Here's how the part is built. I have some questions about the finished solid (model axes, mm). A direction names the side the tool comes from. Give positions to 0.01 mm unless a question says otherwise; leave off trailing zeros. Loops run counter-clockwise (first coordinate to the right, second up) from the corner with the lowest first, then second, coordinate; pieces in that order, holes last. Notation, with made-up numbers: (79.25, -39.5) - (138.25, -39.5) arc R24 cw to (138.25, -6.5) - close; hole circle Ø8 at (32, 20). An arc over 180 degrees is marked (long way). Use one line per item in the form item = value.
from build123d import *

# Parameters (mm, degrees)
SKETCH1_W           = 34.925
SKETCH1_H           = 25.4
BOSS_EXTRUDE1_DEPTH = 1.5875
BOSS_EXTRUDE2_DEPTH = 4.7625
SKETCH4_W           = 14.2875
SKETCH4_H           = 9.525
BOSS_EXTRUDE7_DEPTH = 6.35
SKETCH6_R           = 1.190625
CUT_EXTRUDE1_DEPTH  = 24.759524406


with BuildPart() as part:
    # Sketch1 → Boss-Extrude1 (new body)
    with BuildSketch(Plane(origin=(0, 0, 0), x_dir=(1, 0, 0), z_dir=(0, 1, 0))):
        Rectangle(SKETCH1_W, SKETCH1_H)
    extrude(amount=BOSS_EXTRUDE1_DEPTH)

    # Sketch2 → Boss-Extrude2 (add)
    with BuildSketch(Plane(origin=(0, 1.5875, 0), x_dir=(1, 0, 0), z_dir=(0, 1, 0))):
        Polygon((-4.7625, 11.1125), (11.1125, 11.1125), (11.1125, 6.35), (17.4625, 6.35), (17.4625, -6.35), (11.1125, -6.35), (11.1125, -11.1125), (-4.7625, -11.1125), align=None)
    extrude(amount=BOSS_EXTRUDE2_DEPTH)

    # Sketch4 → Boss-Extrude7 (add)
    with BuildSketch(Plane(origin=(0, 1.5875, 0), x_dir=(1, 0, 0), z_dir=(0, 1, 0))):
        with Locations((-11.90625, 0)):
            Rectangle(SKETCH4_W, SKETCH4_H)
    extrude(amount=BOSS_EXTRUDE7_DEPTH)

    # Sketch6 → Cut-Extrude1 (cut, through all)
    with BuildSketch(Plane(origin=(0, 1.5875, 0), x_dir=(1, 0, 0), z_dir=(0, 1, 0))):
        with Locations(Location((-15.875, 11.1125, 0), (0, 0, 270))):
            Circle(SKETCH6_R)
        with Locations(Location((-15.875, -11.1125, 0), (0, 0, 270))):
            Circle(SKETCH6_R)
        with Locations(Location((15.875, -11.1125, 0), (0, 0, 270))):
            Circle(SKETCH6_R)
        with Locations(Location((15.875, 11.1125, 0), (0, 0, 270))):
            Circle(SKETCH6_R)
    extrude(amount=-CUT_EXTRUDE1_DEPTH, mode=Mode.SUBTRACT)


solid = part.part
(1) If I drill on probe 1 along Y at (x, z) = (4, 6.25); probe 2 along Z at (x, y) = (0, 5.5); probe 3 along X at (y, z) = (7.5, -4.5), over which ranges is the centre line in solid material (lowest first)?
Geometry says:
probe_1 = 0 to 6.35
probe_2 = -11.11 to 11.11
probe_3 = -19.05 to -4.76
(2) For faces 1 (the flat face through (14, 4, -6.35)), 2 (the flat face through (-17.462, 1, 0)), 3 (the flat face through (3, 4, -11.112)), which set-ups out of +Z, -Z, +X, -X, +Y, -Y let a thin tool reach every point of the face, with its end or its side?
Geometry says:
face_1 = -Z, +X, +Y
face_2 = +Z, -Z, -X, -Y
face_3 = -Z, +X, -X, +Y
(3) For P1, Ø1.3, axis at x = -18, z = -2, coming from the -Y side; P2, Ø4, axis at y = 4.5, z = -8.5, coming from the +X side; P3, Ø3, axis at x = 15.88, z = 11.11, coming from the +Y side; P4, Ø4, axis at x = 5.5, z = -7.5, coming from the +Y side, each with a flat end and sliding along its axis, tell me the tip position at first contact or that it passes through.
Geometry says:
P1 = 0
P2 = 11.11
P3 = 1.59
P4 = 6.35
(4) Thinking about a two-plate mould opening in Z: for faces 4 (the flat face through (0, 1, 12.7)), 5 (the cylindrical face through (17.055, 0.805, 10.958)), 6 (the flat face through (-12, 5, -4.762)), which applies, pulls with the +Z half, pulls with the -Z half, needs draft (parallel to the pull), parting line crosses it, or undercut?
Geometry says:
face_4 = pulls with the +Z half
face_5 = undercut
face_6 = pulls with the -Z half
(5) If we section it at C-C (y = 5): List the corners of the cut face in (x, z) for me.
Geometry says:
outline = (-19.05, -4.76) - (-4.76, -4.76) - (-4.76, -11.11) - (11.11, -11.11) - (11.11, -6.35) - (17.46, -6.35) - (17.46, 6.35) - (11.11, 6.35) - (11.11, 11.11) - (-4.76, 11.11) - (-4.76, 4.76) - (-19.05, 4.76) - close
(6) If we section it at D-D (x = 15.5): List the corners of the cut face in (y, z) for me.
Geometry says:
outline = (0, -12.7) - (1.59, -12.7) - (1.59, -12.24) - (0, -12.24) - close; (0, -9.98) - (1.59, -9.98) - (1.59, -6.35) - (6.35, -6.35) - (6.35, 6.35) - (1.59, 6.35) - (1.59, 9.98) - (0, 9.98) - close; (0, 12.24) - (1.59, 12.24) - (1.59, 12.7) - (0, 12.7) - close
(7) If we section it at B-B (z = -8.25): List the corners of the cut face in (x, y) for me.
Geometry says:
outline = (-17.46, 0) - (17.46, 0) - (17.46, 1.59) - (11.11, 1.59) - (11.11, 6.35) - (-4.76, 6.35) - (-4.76, 1.59) - (-17.46, 1.59) - close
(8) If we section it at A-A (x = 5.5): List the corners of the cut face in (y, z) for me.
Geometry says:
outline = (0, -12.7) - (1.59, -12.7) - (1.59, -11.11) - (6.35, -11.11) - (6.35, 11.11) - (1.59, 11.11) - (1.59, 12.7) - (0, 12.7) - close
